CAD build for the part. Positions are in the model's coordinates, mm. A direction names the side the tool comes from. Give positions to 0.01 mm unless a question says otherwise; leave off trailing zeros. Write each loop counter-clockwise with the first axis right and the second up, starting at its lowest first coordinate (ties: lowest second). Pieces come first, ordered by that corner, then holes. Notation, with made-up numbers: (-20.75, 65) - (-5.75, 65) arc R7 cw to (-5.75, 69) - close; hole circle Ø8 at (42.25, 72). An arc over 180 degrees is marked (long way). Put each result on its own line as item: value. Start each with the question number.
1. Wall check: line 1 (X direction, y = 19.3, z = -7.15); line 2 (Y direction, x = -16.5, z = -5); line 3 (Y direction, x = -1, z = 4). Give the ranges that are in metal, low to high.
2. Cut at A-A on x = 16. List the corners of the cut face in (y, z).
3. Drop flat-ended pins along their axis: pin 1 (10 mm diameter, centred on y = -11, z = 13, fed in from -X); pin 2 (4 mm diameter, centred on x = 6.93, z = 7.85, fed in from -Y); pin 3 (3 mm diameter, centred on x = -13.07, z = -7.15, fed in from +Y). Give the stop position or say it passes through.
4. Mould opens along Y. For faces 5 (the flat face through (0, -61, 0)), 6 (the flat face through (17, -12, 0)), 7 (the flat face through (20, -12, 0)) say: +Y half, -Y half, draft (parallel to the pull), parting line (faces both ways), or undercut.
5. Cut at C-C on z = -7.15. List the corners of the cut face in (x, y).
6. Cut at D-D on x = -13. List the corners of the cut face in (y, z), and give its area (3 significant figures).
7. Tool access for faces 1 (the flat face through (-9, -43, 0)), 2 (the cylindrical face through (-13.44, 18.52, 9.51)), 3 (the flat face through (-1, 17, 0)), 4 (the flat face through (-20, -42, 0)): list every direction of +Z, -Z, +X, -X, +Y, -Y with a clear straight run to the whole face (end or side of a thin tool).
8. Cut at B-B on z = 12.5. List the corners of the cut face in (x, y).
from build123d import *

# Parameters (mm, degrees)
BOSS_EXTRUDE1_DEPTH       = 25
SKETCH3_R                 = 8
BOSS_EXTRUDE2_DEPTH       = 18
M3_CLEARANCE_HOLE1_REACH  = 89.098
M3_CLEARANCE_HOLE1_BORE_R = 1.7


with BuildPart() as part:
    # Sketch2 → Boss-Extrude1 (new, symmetric)
    with BuildSketch(Plane.XY):
        Polygon((-20, 20), (20, 20), (20, -40), (20, -43), (-20, -43), (-20, -40), (17, -40), (17, 17), (-20, 17), align=None)
    extrude(amount=BOSS_EXTRUDE1_DEPTH, both=True)

    # Sketch3 → Boss-Extrude2 (add)
    with BuildSketch(Plane.XZ.offset(43)):
        Circle(SKETCH3_R)
    extrude(amount=BOSS_EXTRUDE2_DEPTH)

    # M3 Clearance Hole1 bore → M3 Clearance Hole1 (cut, up to next)
    with BuildSketch(Plane(origin=(0, 20, 0), x_dir=(1, 0, 0), z_dir=(0, 1, 0)), mode=Mode.PRIVATE) as m3_clearance_hole1_sk1:
        with Locations((-13.072595628, -7.85)):
            Circle(M3_CLEARANCE_HOLE1_BORE_R)
    m3_clearance_hole1_tool1 = extrude(m3_clearance_hole1_sk1.sketch, amount=-M3_CLEARANCE_HOLE1_REACH, mode=Mode.PRIVATE) & part.part
    # M3 Clearance Hole1 bore → M3 Clearance Hole1 (cut, up to next)
    with BuildSketch(Plane(origin=(0, 20, 0), x_dir=(1, 0, 0), z_dir=(0, 1, 0)), mode=Mode.PRIVATE) as m3_clearance_hole1_sk2:
        with Locations((-13.072595628, 7.15)):
            Circle(M3_CLEARANCE_HOLE1_BORE_R)
    m3_clearance_hole1_tool2 = extrude(m3_clearance_hole1_sk2.sketch, amount=-M3_CLEARANCE_HOLE1_REACH, mode=Mode.PRIVATE) & part.part
    # M3 Clearance Hole1 bore → M3 Clearance Hole1 (cut, up to next)
    with BuildSketch(Plane(origin=(0, 20, 0), x_dir=(1, 0, 0), z_dir=(0, 1, 0)), mode=Mode.PRIVATE) as m3_clearance_hole1_sk3:
        with Locations((6.927404372, -7.85)):
            Circle(M3_CLEARANCE_HOLE1_BORE_R)
    m3_clearance_hole1_tool3 = extrude(m3_clearance_hole1_sk3.sketch, amount=-M3_CLEARANCE_HOLE1_REACH, mode=Mode.PRIVATE) & part.part
    # M3 Clearance Hole1 bore → M3 Clearance Hole1 (cut, up to next)
    with BuildSketch(Plane(origin=(0, 20, 0), x_dir=(1, 0, 0), z_dir=(0, 1, 0)), mode=Mode.PRIVATE) as m3_clearance_hole1_sk4:
        with Locations((6.927404372, 7.15)):
            Circle(M3_CLEARANCE_HOLE1_BORE_R)
    m3_clearance_hole1_tool4 = extrude(m3_clearance_hole1_sk4.sketch, amount=-M3_CLEARANCE_HOLE1_REACH, mode=Mode.PRIVATE) & part.part
    add(m3_clearance_hole1_tool1.solids().sort_by_distance((-13.072596, 20, 7.85))[0], mode=Mode.SUBTRACT)
    add(m3_clearance_hole1_tool2.solids().sort_by_distance((-13.072596, 20, -7.15))[0], mode=Mode.SUBTRACT)
    add(m3_clearance_hole1_tool3.solids().sort_by_distance((6.927404, 20, 7.85))[0], mode=Mode.SUBTRACT)
    add(m3_clearance_hole1_tool4.solids().sort_by_distance((6.927404, 20, -7.15))[0], mode=Mode.SUBTRACT)


solid = part.part
Report:
1. line 1: x = -20 to -14.77, -11.37 to 5.23, 8.63 to 20
1. line 2: y = -43 to -40, 17 to 20
1. line 3: y = -61 to -40, 17 to 20
2. outline: (-43, -25) - (-40, -25) - (-40, 25) - (-43, 25) - close; (17, -25) - (20, -25) - (20, 25) - (17, 25) - close
3. pin 1: stops at x = 17
3. pin 2: stops at y = -43
3. pin 3: stops at y = -40
4. face 5: -Y half
4. face 6: undercut
4. face 7: draft
5. outline: (-20, -43) - (-3.59, -43) - (-3.59, -61) - (3.59, -61) - (3.59, -43) - (20, -43) - (20, 20) - (8.63, 20) - (8.63, 17) - (17, 17) - (17, -40) - (-20, -40) - close; (-20, 17) - (-14.77, 17) - (-14.77, 20) - (-20, 20) - close; (-11.37, 17) - (5.23, 17) - (5.23, 20) - (-11.37, 20) - close
6. outline: (-43, -25) - (-40, -25) - (-40, 25) - (-43, 25) - close; (17, -25) - (20, -25) - (20, -8.85) - (17, -8.85) - close; (17, -5.45) - (20, -5.45) - (20, 6.15) - (17, 6.15) - close; (17, 9.55) - (20, 9.55) - (20, 25) - (17, 25) - close
6. area: 280 mm²
7. face 1: -Y
7. face 2: +Y
7. face 3: +Z, -Z, -X
7. face 4: +Z, -Z, -X, +Y, -Y
8. outline: (-20, -43) - (20, -43) - (20, 20) - (-20, 20) - (-20, 17) - (17, 17) - (17, -40) - (-20, -40) - close
